Drawing for the job (mm, zero at the part's lowest x, y, z). A direction names the side the tool comes from. Coordinates: 2 decimals unless noted, no trailing zeros. Order: outer loops, then holes, each group sorted by start corner. A loop starts at its lowest first (then second) coordinate and runs counter-clockwise, first axis right, second up.
1) Tool access for the marked faces 4, 5, 6 and 7: list every direction of +Z, -Z, +X, -X, +Y, -Y with a clear straight run to the whole face (end or side of a thin tool).
2) Cut at D-D (y = 11). List the corners of the cut face in (x, z).
3) Pin check, flat tips, straight feed: pin 1 Ø4 at (x, z) = (4.5, 3) entering from +Y; pin 2 Ø1.5 at (x, y) = (11, 16.5) entering from -Z; pin 3 Ø2.5 at (y, z) = (2.5, 2.5) entering from -X (1 decimal). Stop position of each tip, or through.
4) Wall check: L1, parallel to Y at x = 4.5, z = 2.5; L2, parallel to Z at x = 19, y = 2.25; L3, parallel to X at y = 2, z = 8.75 (1 decimal). Give the ranges that are in metal, low to high.
5) Cut at B-B (x = 10.84). List the corners of the cut face in (y, z).
6) Cut at A-A (z = 6.5). List the corners of the cut face in (x, y) (1 decimal).
7) Mould opens along X. For the marked faces 1, 2 and 3 say: +X half, -X half, draft (parallel to the pull), parting line (faces both ways), or undercut.
8) Cut at C-C (y = 2.5). List the corners of the cut face in (x, z) (1 decimal).
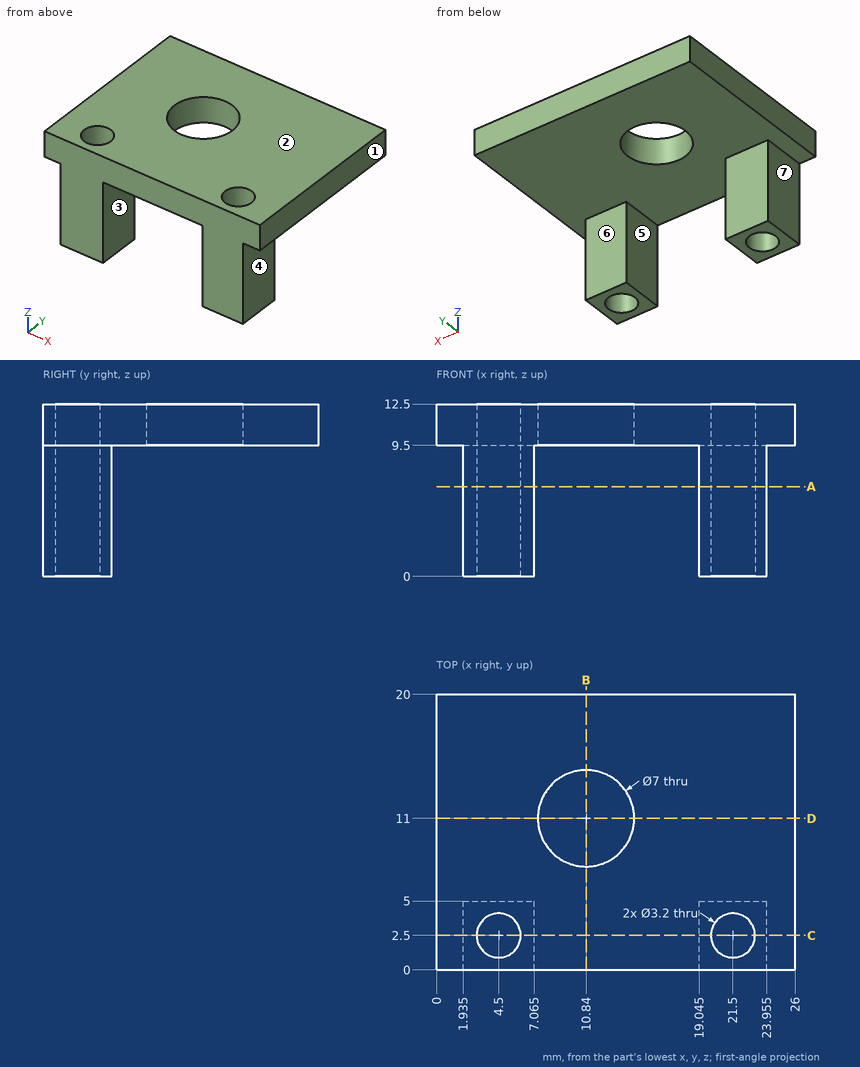
Geometry check:
1. face 4: -Z, +X, +Y, -Y
1. face 5: -Z, +Y, -Y
1. face 6: -Z, +X, -X, +Y
1. face 7: -Z, -X, +Y, -Y
2. outline: (0, 9.5) - (7.34, 9.5) - (7.34, 12.5) - (0, 12.5) - close; (14.34, 9.5) - (26, 9.5) - (26, 12.5) - (14.34, 12.5) - close
3. pin 1: stops at y = 5
3. pin 2: stops at z = 9.5
3. pin 3: stops at x = 1.9
4. L1: y = 0 to 0.9, 4.1 to 5
4. L2: z = 9.5 to 12.5
4. L3: x = 1.9 to 3, 6 to 7.1, 19 to 20, 23 to 24
5. outline: (0, 9.5) - (7.5, 9.5) - (7.5, 12.5) - (0, 12.5) - close; (14.5, 9.5) - (20, 9.5) - (20, 12.5) - (14.5, 12.5) - close
6. outline: (1.9, 0) - (7.1, 0) - (7.1, 5) - (1.9, 5) - close; (19, 0) - (24, 0) - (24, 5) - (19, 5) - close; hole circle Ø3.2 at (4.5, 2.5); hole circle Ø3.2 at (21.5, 2.5)
7. face 1: +X half
7. face 2: draft
7. face 3: undercut
8. outline: (0, 9.5) - (1.9, 9.5) - (1.9, 0) - (2.9, 0) - (2.9, 12.5) - (0, 12.5) - close; (6.1, 0) - (7.1, 0) - (7.1, 9.5) - (19, 9.5) - (19, 0) - (19.9, 0) - (19.9, 12.5) - (6.1, 12.5) - close; (23.1, 0) - (24, 0) - (24, 9.5) - (26, 9.5) - (26, 12.5) - (23.1, 12.5) - close
